The listing builds one solid part. Answer for the finished solid, in the listing's coordinates (mm). A direction names the side the tool comes from. Coordinates: 2 decimals unless noted, no trailing zeros. Order: outer loops, then holes, each group sorted by start corner. A loop starts at its lowest first (then second) coordinate and runs counter-clockwise, first axis right, second up. Notation, with made-up numbers: (43, 55.5) - (71, 55.5) arc R22 ccw to (71, 87.5) - close; hole circle Ø6 at (62.25, -21.75). An arc over 180 degrees is marked (long way). Use one line per item in the form item = value. Start each with the question number.
Item 1: Section B-B, the plane z = -2.75 is taken. Write down the section's boundary in (x, y).
Item 2: Consider line 1 along Y through (x, z) = (6, -1.75); line 2 along Y through (x, z) = (19, -1); line 3 along Y through (x, z) = (26.5, 0.75). Determine where each line is inside the solid, lowest interval first. Write a range as [from, to].
Item 3: A tool of negligible diameter and unlimited length cuts with its end or side. For faces 1 (the cylindrical face through (-0.802, 3.612, -3.014)), 2 (the cylindrical face through (25.366, 9.035, -2.056)), 3 (the flat face through (29.314, 19.889, -4.028)), from which of +Z, -Z, +X, -X, +Y, -Y can it reach the whole face along a straight path? Write none if from no direction.
Item 4: Each of these flat-tipped pins is pushed along its axis until it touches: pin 1 Ø11.5 at (x, y) = (16, 18.5) entering from -Z; pin 2 Ø2.5 at (x, y) = (40.61, 21.6) entering from +Z; pin 3 Ø2 at (y, z) = (19.5, -3.5) entering from -X; pin 4 Ø9 at (x, y) = (8, 2.5) entering from -Z. Where does it stop, or does it pass through?
Item 5: Section A-A, the plane x = 0 is taken. Write down the section's boundary in (y, z).
Item 6: Section C-C, the plane y = 22.5 is taken. Write down the section's boundary in (x, z), and give its area (3 significant figures).
Item 7: Section D-D, the plane z = -0.25 is taken. Write down the section's boundary in (x, y).
Item 8: The mould has two halves that part along X. Classify faces 4 (the flat face through (15, -0.67, -0.03)), 5 (the flat face through (8.3, 19.9, -4)), 6 (the cylindrical face through (32.15, 16.15, -2.06)), 7 (the cylindrical face through (23.1, 16.9, 0)): released by +X, released by -X, zero draft, split by the parting line, or undercut.
from build123d import *

# Parameters (mm, degrees)
BOSS_EXTRUDE1_DEPTH      = 2
BOSS_EXTRUDE1_DEPTH_BACK = 2
SKETCH2_R                = 1.7
FILLET1_R                = 20
BOSS_EXTRUDE4_START      = 4
SKETCH7_R                = 1.7
BOSS_EXTRUDE4_DEPTH      = 4
BOSS_EXTRUDE5_START      = 2
SKETCH8_R                = 3.7
SKETCH8_R_2              = 1.7
BOSS_EXTRUDE5_DEPTH      = 2
FILLET4_R                = 2
SKETCH9_R                = 1.7
CUT_EXTRUDE1_DEPTH       = 55.759144692


with BuildPart() as part:
    # Sketch2 → Boss-Extrude1 (new, two sides: drawn at the far end of the back side and taken through both)
    with BuildSketch(Plane.XY.offset(-BOSS_EXTRUDE1_DEPTH_BACK)):
        with BuildLine():
            Line((1.575752274, -4.745208612), (34.456924853, 5.232629629))
            Line((34.456924853, 5.232629629), (44.296635241, 16.864742156))
            ThreePointArc((44.296635241, 16.864742156), (46.218376178, 23.740514028), (40.203783054, 27.586810508))
            Line((40.203783054, 27.586810508), (7.512886707, 26.600773906))
            ThreePointArc((7.512886707, 26.600773906), (2.79322071, 19.950091357), (10.629154827, 17.690675057))
            Line((10.629154827, 17.690675057), (25.733767379, 18.146266751))
            Line((25.733767379, 18.146266751), (18.728666276, 9.86511608))
            Line((18.728666276, 9.86511608), (1.70658462, 4.699741369))
            ThreePointArc((1.70658462, 4.699741369), (-4.999520368, 0.069253832), (1.575752274, -4.745208612))
        make_face()
        Circle(SKETCH2_R, mode=Mode.SUBTRACT)
        with Locations((40.612886707, 21.600773906)):
            Circle(SKETCH2_R, mode=Mode.SUBTRACT)
        with Locations((7.512886707, 21.600773906)):
            Circle(SKETCH2_R, mode=Mode.SUBTRACT)
    extrude(amount=BOSS_EXTRUDE1_DEPTH + BOSS_EXTRUDE1_DEPTH_BACK)

    # Fillet1
    fillet1_edges = [part.edges().sort_by_distance(p)[0] for p in [
        (34.456924853, 5.232629629, 0),
        (18.728666276, 9.86511608, 0),
    ]]
    fillet(fillet1_edges, radius=FILLET1_R)

    # Sketch7 → Boss-Extrude4 (add)
    with BuildSketch(Plane(origin=(0, 0, -2), x_dir=(-1, 0, 0), z_dir=(0, 0, -1)).offset(BOSS_EXTRUDE4_START)):
        with BuildLine():
            Line((-36.733417778, 26.177860406), (-21.683989193, 13.422192867))
            ThreePointArc((-21.683989193, 13.422192867), (-21.70362245, 5.922427438), (-28.807655282, 3.518350802))
            ThreePointArc((-28.807655282, 3.518350802), (-33.988212002, 5.945467438), (-38.269694349, 9.739933408))
            Line((-38.269694349, 9.739933408), (-44.296635241, 16.864742156))
            ThreePointArc((-44.296635241, 16.864742156), (-45.270474012, 25.383217626), (-36.733417778, 26.177860406))
        make_face()
        with Locations(Location((-40.612886707, 21.600773906, 0), (0, 0, 180))):
            Circle(SKETCH7_R, mode=Mode.SUBTRACT)
    extrude(amount=-BOSS_EXTRUDE4_DEPTH)

    # Sketch8 → Boss-Extrude5 (add)
    # profile 1 of 2: a face of its own
    with BuildSketch(Plane(origin=(0, 0, -2), x_dir=(-1, 0, 0), z_dir=(0, 0, -1)).offset(BOSS_EXTRUDE5_START)):
        with Locations(Location((-7.512886707, 21.600773906, 0), (0, 0, 180))):
            Circle(SKETCH8_R)
        with Locations(Location((-7.512886707, 21.600773906, 0), (0, 0, 180))):
            Circle(SKETCH8_R_2, mode=Mode.SUBTRACT)
    # profile 2 of 2: a face of its own
    with BuildSketch(Plane(origin=(0, 0, -2), x_dir=(-1, 0, 0), z_dir=(0, 0, -1)).offset(BOSS_EXTRUDE5_START)):
        with Locations(Location((0, 0, 0), (0, 0, 180))):
            Circle(SKETCH8_R)
        with Locations(Location((0, 0, 0), (0, 0, 180))):
            Circle(SKETCH8_R_2, mode=Mode.SUBTRACT)
    extrude(amount=-BOSS_EXTRUDE5_DEPTH)

    # Fillet4
    fillet4_edges = [part.edges().sort_by_distance(p)[0] for p in [
        (25.733767379, 18.146266751, 0),
    ]]
    fillet(fillet4_edges, radius=FILLET4_R)

    # Sketch9 → Cut-Extrude1 (cut, through all)
    with BuildSketch(Plane(origin=(0, 0, -6), x_dir=(-1, 0, 0), z_dir=(0, 0, -1))):
        with Locations((-33.774027465, 15.643013901)):
            Circle(SKETCH9_R)
        with Locations((-26.936063231, 9.686033593)):
            Circle(SKETCH9_R)
    extrude(amount=-CUT_EXTRUDE1_DEPTH, mode=Mode.SUBTRACT)


solid = part.part
Response:
q1.outline = circle Ø7.4 at (0, 0); circle Ø7.4 at (7.51, 21.6); (21.68, 13.42) arc R6.45 ccw to (28.81, 3.52) arc R20 ccw to (38.27, 9.74) - (44.3, 16.86) arc R6 ccw (long way) to (36.73, 26.18) - close; hole circle Ø3.4 at (0, 0); hole circle Ø3.4 at (7.51, 21.6); hole circle Ø3.4 at (26.94, 9.69); hole circle Ø3.4 at (33.77, 15.64); hole circle Ø3.4 at (40.61, 21.6)
q2.line_1 = [-3.4, 6], [16.84, 20.83], [22.38, 26.37]
q2.line_2 = [0.54, 11.09], [17.94, 26.95]
q2.line_3 = [2.82, 8.04], [11.33, 27.17]
q3.face_1 = -Z
q3.face_2 = +Z, -Z
q3.face_3 = -Z, +Y
q4.pin_1 = -4
q4.pin_2 = through
q4.pin_3 = 3.98
q4.pin_4 = -2
q5.outline = (-5, -2) - (-3.7, -2) - (-3.7, -4) - (-1.7, -4) - (-1.7, 2) - (-5, 2) - close; (1.7, -4) - (3.7, -4) - (3.7, -2) - (5, -2) - (5, 2) - (1.7, 2) - close
q6.outline = (2.59, -2) - (3.92, -2) - (3.92, -4) - (6.07, -4) - (6.07, 2) - (2.59, 2) - close; (8.96, -4) - (11.1, -4) - (11.1, -2) - (32.39, -2) - (32.39, -6) - (39.17, -6) - (39.17, 2) - (8.96, 2) - close; (42.06, -6) - (46.55, -6) - (46.55, 2) - (42.06, 2) - close
q6.area = 206 mm2
q7.outline = (1.58, -4.75) - (28.81, 3.52) arc R20 ccw to (38.27, 9.74) - (44.3, 16.86) arc R6 ccw to (40.2, 27.59) - (7.51, 26.6) arc R5 ccw (long way) to (10.63, 17.69) - (21.25, 18.01) arc R2 cw to (22.84, 14.72) - (22.54, 14.37) arc R20 cw to (13.08, 8.15) - (1.71, 4.7) arc R5 ccw (long way) to start; hole circle Ø3.4 at (0, 0); hole circle Ø3.4 at (7.51, 21.6); hole circle Ø3.4 at (26.94, 9.69); hole circle Ø3.4 at (33.77, 15.64); hole circle Ø3.4 at (40.61, 21.6)
q8.face_4 = released by +X
q8.face_5 = zero draft
q8.face_6 = undercut
q8.face_7 = undercut
